The listing builds one solid part. Answer for the finished solid, in the listing's coordinates (mm). A direction names the side the tool comes from. Coordinates: 2 decimals unless noted, no trailing zeros. Write each loop counter-clockwise with the first axis right and the second up, starting at its lowest first coordinate (ties: lowest second). Pieces come first, ordered by that corner, then holes.
```python
from build123d import *

# Parameters (mm, degrees)
SKETCH_W     = 50
SKETCH_H     = 12
SKETCH_R     = 1.2
PAD_DEPTH    = 1.5
SKETCH001_W  = 10
SKETCH001_H  = 12
PAD001_DEPTH = 3.5
POCKET_DEPTH = 10
FILLET_R     = 2


with BuildPart() as part:
    # Sketch → Pad (new body)
    with BuildSketch(Plane.XY):
        Rectangle(SKETCH_W, SKETCH_H)
        with Locations((-20, 0)):
            Circle(SKETCH_R, mode=Mode.SUBTRACT)
        with Locations((20, 0)):
            Circle(SKETCH_R, mode=Mode.SUBTRACT)
    extrude(amount=PAD_DEPTH)

    # Sketch001 (on Face8 of Pad) → Pad001 (join)
    with BuildSketch(Plane.XY.offset(1.5)):
        Rectangle(SKETCH001_W, SKETCH001_H)
    extrude(amount=PAD001_DEPTH)

    # Sketch002 (on Face12 of Pad001) → Pocket (cut)
    with BuildSketch(Plane.YZ.offset(5)):
        Polygon((3, 1.5), (3, 3.5), (-4.5, 3.5), (-4.5, 2.5), (-6, 2.5), (-6, 1.5), align=None)
    extrude(amount=-POCKET_DEPTH, mode=Mode.SUBTRACT)

    # Fillet
    fillet_edges = [part.edges().sort_by_distance(p)[0] for p in [
        (25, -6, 0.75),
        (25, 6, 0.75),
        (-25, -6, 0.75),
        (-25, 6, 0.75),
    ]]
    fillet(fillet_edges, radius=FILLET_R)


solid = part.part
```
(1) Section C-C, the plane y = 0 is taken. Write down the section's boundary in (x, z), plus the area to 3 significant figures.
(2) Each of these flat-tipped pins is pushed along its axis until it touches: pin 1 (1.8 mm diameter, centred on y = 0.5, z = 3, fed in from +X); pin 2 (3 mm diameter, centred on x = 20, y = 0, fed in from +Z); pin 3 (3 mm diameter, centred on x = 16.5, z = 4.5, fed in from -Y); pin 4 (1.5 mm diameter, centred on y = 2.5, z = 3.5, fed in from -X). Where does it stop, or does it pass through?
(3) Section A-A, the plane z = 2.95 is taken. Write down the section's boundary in (x, y).
(4) Find the intervals of material crossed by probe 1 along Z at (x, y) = (-2, -4); probe 2 along Y at (x, z) = (-20, 0.95); probe 3 along Z at (x, y) = (-8.5, 0.25), in increasing order.
(5) Section B-B, the plane x = 20 is taken. Write down the section's boundary in (y, z).
(6) For a pull along Y with two mould halves and no side action, classify faces 4 (the cylindrical face through (18.8, 0.05, 0.74)), 5 (the flat face through (-25, 0, 1)), 6 (the flat face through (0, -6, 1)) as pulls with the +Y half, pulls with the -Y half, needs draft (parallel to the pull), parting line crosses it, or undercut.
(7) Section D-D, the plane x = -1.5 is taken. Write down the section's boundary in (y, z), plus the area to 3 significant figures.
(8) Which of the six approach directions +Z, -Z, +X, -X, +Y, -Y give full straight-line access (tool end or side, diameter ignored) to faces 1 (the flat face through (0, 3, 2)), 2 (the flat face through (0, -5, 2.5)), 3 (the flat face through (-5, 1, 4))?
Solution:
1. outline: (-25, 0) - (-21.2, 0) - (-21.2, 1.5) - (-25, 1.5) - close; (-18.8, 0) - (18.8, 0) - (18.8, 1.5) - (-18.8, 1.5) - close; (-5, 3.5) - (5, 3.5) - (5, 5) - (-5, 5) - close; (21.2, 0) - (25, 0) - (25, 1.5) - (21.2, 1.5) - close
1. area: 82.8 mm2
2. pin 1: stops at x = 5
2. pin 2: stops at z = 1.5
2. pin 3: passes through
2. pin 4: stops at x = -5
3. outline: (-5, -6) - (5, -6) - (5, -4.5) - (-5, -4.5) - close; (-5, 3) - (5, 3) - (5, 6) - (-5, 6) - close
4. probe 1: z = 0 to 1.5, 3.5 to 5
4. probe 2: y = -6 to -1.2, 1.2 to 6
4. probe 3: z = 0 to 1.5
5. outline: (-6, 0) - (-1.2, 0) - (-1.2, 1.5) - (-6, 1.5) - close; (1.2, 0) - (6, 0) - (6, 1.5) - (1.2, 1.5) - close
6. face 4: undercut
6. face 5: needs draft
6. face 6: pulls with the -Y half
7. outline: (-6, 0) - (6, 0) - (6, 5) - (-6, 5) - (-6, 2.5) - (-4.5, 2.5) - (-4.5, 3.5) - (3, 3.5) - (3, 1.5) - (-6, 1.5) - close
7. area: 43.5 mm2
8. face 1: +X, -X
8. face 2: +X, -X, -Y
8. face 3: +Z, -X, +Y, -Y
